Check sheet for the modelled part. Datum: model origin and axes. Units: mm. Give positions to 0.01 mm unless a question says otherwise; leave off trailing zeros. Write each loop counter-clockwise with the first axis right and the second up, starting at its lowest first coordinate (ties: lowest second). Pieces come first, ordered by that corner, then holes. Notation, with made-up numbers: M 63.5,26 L 122.5,26 A6 cw 122.5,30 Z; hole C -32.5,79.25 d1. An arc over 180 degrees is marked long. Use CSV: the item, a comma, the result in double quotes. Start each with the question number.
1. Cross-section at B-B, the plane x = -113. Enter the section's corners in (y, z), and give its area (3 significant figures).
2. Cross-section at C-C, the plane z = 2. State how many separate pieces and enclosed holes the cut face has, and give its area (3 significant figures).
3. Cross-section at A-A, the plane y = -0.5. Enter the section's corners in (x, z).
4. Depth check by flat-ended pin: P1, Ø0.9, axis at x = 48.5, z = 2, coming from the +Y side; P2, Ø0.9, axis at x = -129.5, z = 1.5, coming from the -Y side; P3, Ø0.9, axis at y = -10, z = 1, coming from the -X side. Enter the tip coordinate at first touch or a pass-through.
5. Scan lines: line 1 (Y direction, x = 91.5, z = 1.2); line 2 (X direction, y = 6.5, z = 0.9); line 3 (X direction, y = -6.75, z = 0.8). Record each from-to range of solid material in increasing order.
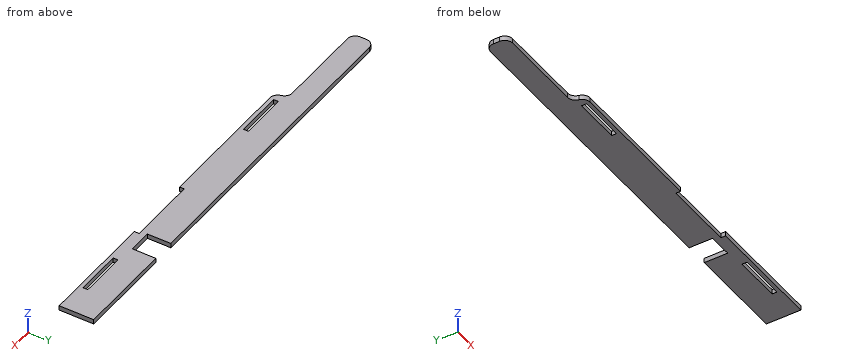
Autodesk Inventor part; units mm, degrees
ref_plane "YZ Plane" through (0, 0, 0) normal (1, 0, 0) x (0, 1, 0)
ref_plane "XZ Plane" through (0, 0, 0) normal (0, 1, 0) x (-1, 0, 0)
ref_plane "XY Plane" through (0, 0, 0) normal (0, 0, 1) x (1, 0, 0)
sketch "Sketch1" plane through (0, 0, 0) normal (0, 0, 1) x (1, 0, 0)
  line L0 (-120, -11) -> (120, -11)
  line L1 (120, -11) -> (120, 11)
  line L2 (120, 11) -> (-120, 11)
  line L3 (-120, 11) -> (-120, -11)
  line L4 (-120, -11) -> (120, 11) construction
  line L5 (120, -11) -> (-120, 11) construction
  line L6 (-90, -5.43) -> (-59.93, -5.43)
  line L7 (-59.93, -5.43) -> (-59.93, -8.5)
  line L8 (-59.93, -8.5) -> (-90, -8.5)
  line L9 (-90, -8.5) -> (-90, -5.43)
  line L10 (-90, -5.43) -> (-59.93, -8.5) construction
  line L11 (-59.93, -5.43) -> (-90, -8.5) construction
  line L12 (100.14, -5.42) -> (70.07, -5.42)
  line L13 (70.07, -5.42) -> (70.07, -8.5)
  line L14 (70.07, -8.5) -> (100.14, -8.5)
  line L15 (100.14, -8.5) -> (100.14, -5.42)
  line L16 (100.14, -5.42) -> (70.07, -8.5) construction
  line L17 (70.07, -5.42) -> (100.14, -8.5) construction
  line L18 (-120, -11) -> (-95, -11)
  line L19 (-95, -11) -> (-95, -3)
  line L20 (-95, -3) -> (-120, -3)
  line L21 (-120, -3) -> (-120, -11)
  line L22 (43, 11) -> (58, 11)
  line L23 (58, 11) -> (58, -4)
  line L24 (58, -4) -> (43, -4)
  line L25 (43, -4) -> (43, 11)
  line L26 (-120, 11) -> (-160, 11)
  line L27 (-160, 11) -> (-160, -3)
  line L28 (-160, -3) -> (-120, -3)
  line L29 (-120, -3) -> (-120, 11)
  point P0 (0, 0)
  point P1 (0, 0)
  point P2 (-74.965, -6.965)
  point P3 (85.105, -6.96)
  point P4 (58, 11)
  point P5 (-140, -3)
  dimension "d0" = 240
  dimension "d1" = 22
  dimension "d2" = 30.07
  dimension "d3" = 3.07
  dimension "d4" = 2.5
  dimension "d5" = 30
  dimension "d6" = 30.07
  dimension "d7" = 3.08
  dimension "d8" = 2.5
  dimension "d9" = 130
  dimension "d10" = 25
  dimension "d11" = 8
  dimension "d12" = 15
  dimension "d13" = 15
  dimension "d14" = 43
  dimension "d17" = 40
extrude "Plate1" add sketch "Sketch1" along normal blind 3 contours L19 L20 L3 L2 L25 L24 L23 L1 L0 | L28 L27 L26 L3
fillet "Corner Round1" radius 5 4 edges at (-95, -3, 1.5) (-95, -11, 1.5) (-160, -3, 1.5) (-160, 11, 1.5)
sketch "Sketch3" plane through (0, 0, 3) normal (0, 0, 1) x (1, 0, 0)
  line L0 (-90.202, -11) -> (120, -11)
  line L1 (0, -11) -> (45, -11)
  line L2 (45, -11) -> (45, -8)
  line L3 (45, -8) -> (0, -8)
  line L4 (0, -8) -> (0, -11)
  point P0 (0, 0)
  dimension "d22" = 3
  dimension "d23" = 45
extrude "Cut2" cut sketch "Sketch3" against normal blind 3
equation "\"d24\" = Thickness"
equation "\"d15\" = Thickness"
equation "\"BendRadius\" = Thickness"
equation "\"BendReliefWidth\" = Thickness"
equation "\"BendReliefDepth\" = 0.5 * Thickness"
equation "\"CornerReliefSize\" = 4 * Thickness"
equation "\"MinimumRemnant\" = 2 * Thickness"
equation "\"TransitionRadius\" = BendRadius"
equation "\"JacobiRadiusSize\" = BendRadius"
equation "\"GapSize\" = Thickness"
properties part number "Starting Path Wall ( Servo )"
Worked answers:
1,outline,"M -3,0 L 11,0 L 11,3 L -3,3 Z"
1,area,"42.0 mm^2"
2,separate pieces,"1"
2,enclosed holes,"2"
2,area,"5,090 mm^2"
3,outline,"M -159.33,0 L 43,0 L 43,3 L -159.33,3 Z; M 58,0 L 120,0 L 120,3 L 58,3 Z"
4,P1,"stops at y = -4"
4,P2,"stops at y = -3"
4,P3,"stops at x = -93.72"
5,line 1,"y = -11 to -8.5, -5.42 to 11"
5,line 2,"x = -159.97 to 43, 58 to 120"
5,line 3,"x = -95.16 to -90, -59.93 to 70.07, 100.14 to 120"
